Autodesk Inventor part; units mm, degrees
ref_plane "YZ Plane" through (0, 0, 0) normal (1, 0, 0) x (0, 1, 0)
ref_plane "XZ Plane" through (0, 0, 0) normal (0, 1, 0) x (-1, 0, 0)
ref_plane "XY Plane" through (0, 0, 0) normal (0, 0, 1) x (1, 0, 0)
sketch "Sketch1" plane through (0, 0, 0) normal (0, 0, 1) x (1, 0, 0)
  line L0 (-19.0052, 9.318) -> (0.9948, 9.318)
  line L1 (0.9948, 9.318) -> (0.9948, -10.682)
  line L2 (0.9948, -10.682) -> (-19.0052, -10.682)
  line L3 (-19.0052, -10.682) -> (-19.0052, 9.318)
  circle A0 centre (-17.0052, 4.5395) radius 1.5
  circle A1 centre (-1.0052, 4.5395) radius 1.5
  dimension "d1" = 20
  dimension "d2" = 20
  dimension "d3" = 3
  dimension "d4" = 2
extrude "Extrusion1" add sketch "Sketch1" along normal blind 1
sketch "Sketch2" plane through (0, 0, 1) normal (0, 0, 1) x (1, 0, 0)
  circle A0 centre (-13.5052, 2.318) radius 1
  circle A1 centre (-10.5052, 2.318) radius 1
  circle A2 centre (-17.0052, 4.5395) radius 1.5
  circle A3 centre (-1.0052, 4.5395) radius 1.5
  line L0 (0.9948, 9.318) -> (-19.0052, 9.318)
  line L1 (-9.0052, 9.318) -> (-9.0052, -10.5627)
  circle A4 centre (-4.5052, 2.318) radius 1
  circle A5 centre (-7.5052, 2.318) radius 1
  point P0 (0, 0)
  point P1 (-12.2352, 2.318)
  point P2 (-5.7752, 2.318)
  dimension "d7" = 2
  dimension "d8" = 2
  dimension "d11" = 3
  dimension "d14" = 3.5
  dimension "d19" = 7
  dimension "d21" = 7
extrude "Extrusion2" cut sketch "Sketch2" against normal blind 10 contours A0 | A1 | A4 | A5
properties part number "PCB USB-B Hembra"
Input: part model. Units: mm. Frame: model coordinates. Coordinates: 2 decimals unless noted, no trailing zeros. Loops run counter-clockwise (first coordinate to the right, second up) from the corner with the lowest first, then second, coordinate; pieces in that order, holes last.
Q1. Section A-A, the plane x = -17. Return the cut outline in (y, z).
Results are:
outline: (-10.68, 0) - (3.04, 0) - (3.04, 1) - (-10.68, 1) - close; (6.04, 0) - (9.32, 0) - (9.32, 1) - (6.04, 1) - close
Q2. Line query: line 1 along Y through (x, z) = (-17, 0.45); line 2 along X through (y, z) = (3.75, 0.75); line 3 along X through (y, z) = (5, 0.45). Output: solid intervals per line, ascending.
Results are:
line 1: y = -10.68 to 3.04, 6.04 to 9.32
line 2: x = -19.01 to -18.28, -15.73 to -2.28, 0.27 to 0.99
line 3: x = -19.01 to -18.43, -15.58 to -2.43, 0.42 to 0.99
Q3. Section C-C, the plane x = -10.75. Return the cut outline in (y, z).
Results are:
outline: (-10.68, 0) - (1.35, 0) - (1.35, 1) - (-10.68, 1) - close; (3.29, 0) - (9.32, 0) - (9.32, 1) - (3.29, 1) - close
Q4. Mould query, pull axis X, two halves, no side actions, for faces 1 (the flat face through (-8.9, -10.682, 0.5)), 2 (the flat face through (-19.005, -0.8, 0.5)), 3 (the cylindrical face through (-9.581, 1.935, 0.507)), 4 (the flat face through (0.995, -0.5, 0.5)). Classes: +X half, -X half, draft (parallel to the pull), parting line (faces both ways), or undercut.
Results are:
face 1: draft
face 2: -X half
face 3: undercut
face 4: +X half
Q5. Contact query for a flat-ended pin moving along its axis: pin 1 (5 mm diameter, centred on x = -1.01, y = 4.54, fed in from -Z). Output: stop coordinate, or through.
Results are:
pin 1: stops at z = 0
Q6. Section B-B, the plane z = 0.15. Return the cut outline in (x, y).
Results are:
outline: (-19.01, -10.68) - (0.99, -10.68) - (0.99, 9.32) - (-19.01, 9.32) - close; hole circle Ø3 at (-17.01, 4.54); hole circle Ø2 at (-13.51, 2.32); hole circle Ø2 at (-10.51, 2.32); hole circle Ø2 at (-7.51, 2.32); hole circle Ø2 at (-4.51, 2.32); hole circle Ø3 at (-1.01, 4.54)
